```python
from build123d import *

# Parameters (mm, degrees)
F0_W     = 7.3944082856
F0_H     = 10
F0_W_2   = 7.394
F0_W_3   = 20
F0_H_2   = 5
F0_W_4   = 12.9295032024
F0_H_3   = 4
F0_W_5   = 4
F0_H_4   = 2
F1_DEPTH = 3


with BuildPart() as f1:
    # F0 (on Top) → F1 (new body)
    with BuildSketch(Plane.XY):
        with BuildLine():
            Line((72.3460563783, -23.3392287046), (-57.1586965515, -23.3392287046))
            Line((-57.1586965515, -23.3392287046), (-57.1586965515, -27.7934716308))
            Line((-57.1586965515, -27.7934716308), (-62.8714114428, -36.0010832548))
            Line((-62.8714114428, -36.0010832548), (-62.8714114428, -86.0010832548))
            ThreePointArc((-62.8714114428, -86.0010832548), (-61.102155393, -91.2274471391), (-56.5220229328, -94.3043828011))
            Line((-56.5220229328, -94.3043828011), (-46.5220229328, -94.3043828011))
            Line((-46.5220229328, -94.3043828011), (-39.6812242775, -101.5984539385))
            Line((-39.6812242775, -101.5984539385), (55.3187757225, -101.5984539385))
            Line((55.3187757225, -101.5984539385), (62.774033672, -94.9336862077))
            Line((62.774033672, -94.9336862077), (72.774033672, -94.9336862077))
            ThreePointArc((72.774033672, -94.9336862077), (76.135356085, -91.3724962002), (77.3572234082, -86.6303866614))
            Line((77.3572234082, -86.6303866614), (77.3572234082, -38.2830989705))
            Line((77.3572234082, -38.2830989705), (72.3460563783, -29.6293018271))
            Line((72.3460563783, -29.6293018271), (72.3460563783, -23.3392287046))
        make_face()
        Polygon((-33.379150033, -48.477938503), (-33.379150033, -46.477938503), (-34.9630750716, -46.477938503), (-34.9630750716, -50.477938503), (-33.379150033, -50.477938503), (-33.379150033, -60.477938503), (-34.9630750716, -60.477938503), (-34.9630750716, -64.477938503), (-33.379150033, -64.477938503), (-33.379150033, -66.477938503), (-49.892578274, -66.477938503), (-49.892578274, -64.477938503), (-47.892578274, -64.477938503), (-47.892578274, -60.477938503), (-49.892578274, -60.477938503), (-49.892578274, -50.477938503), (-47.892578274, -50.477938503), (-47.892578274, -46.477938503), (-49.892578274, -46.477938503), (-49.892578274, -44.477938503), (-45.951873064, -44.477938503), (-45.951873064, -42.477938503), (-47.4065802991, -42.477938503), (-47.4065802991, -40.477938503), (-34.9630750716, -40.477938503), (-31.379150033, -44.477938503), (-31.379150033, -48.477938503), align=None, mode=Mode.SUBTRACT)
        with Locations((-20.7225426286, -55.477938503)):
            Rectangle(F0_W, F0_H, mode=Mode.SUBTRACT)
        with Locations((-9.2900967939, -55.477938503)):
            Rectangle(F0_W_2, F0_H, mode=Mode.SUBTRACT)
        with BuildLine():
            Line((23.9428310841, -64.477938503), (23.9428310841, -36.0010832548))
            Line((23.9428310841, -36.0010832548), (33.941513979, -36.163380414))
            Line((33.941513979, -36.163380414), (33.941513979, -64.477938503))
            ThreePointArc((33.941513979, -64.477938503), (28.9421725316, -69.4772799505), (23.9428310841, -64.477938503))
        make_face(mode=Mode.SUBTRACT)
        with BuildLine():
            Line((38.3750386536, -64.477938503), (38.3750386536, -36.163380414))
            Line((38.3750386536, -36.163380414), (48.3750386536, -36.163380414))
            Line((48.3750386536, -36.163380414), (48.3750386536, -64.477938503))
            ThreePointArc((48.3750386536, -64.477938503), (43.3750386536, -69.477938503), (38.3750386536, -64.477938503))
        make_face(mode=Mode.SUBTRACT)
        with BuildLine():
            ThreePointArc((-28.9360948412, 27.1936530951), (-30.9919428027, 31.9537867139), (-28.9360948412, 36.7139203326))
            ThreePointArc((-28.9360948412, 36.7139203326), (-28.7221124747, 44.6950672996), (-36.7044586735, 44.8582988061))
            Line((-36.7044586735, 44.8582988061), (-62.5819294645, 29.6807988322))
            ThreePointArc((-62.5819294645, 29.6807988322), (-64.9426232399, 21.7216482709), (-57.1586965515, 18.8352252132))
            Line((-57.1586965515, 18.8352252132), (-57.1586965515, 13.1085557863))
            Line((-57.1586965515, 13.1085557863), (-57.1586965515, -11.8914442137))
            Line((-57.1586965515, -11.8914442137), (-57.1586965515, -23.3392287046))
            Line((-57.1586965515, -23.3392287046), (72.3460563783, -23.3392287046))
            Line((72.3460563783, -23.3392287046), (72.3460563783, 20.3706981729))
            ThreePointArc((72.3460563783, 20.3706981729), (77.602081112, 24.9911609789), (74.7467246428, 31.3803246156))
            Line((74.7467246428, 31.3803246156), (48.6460575227, 46.1706990491))
            Line((48.6460575227, 46.1706990491), (48.1593732874, 46.2963732235))
            ThreePointArc((48.1593732874, 46.2963732235), (40.4569849003, 43.1335810056), (42.8548762559, 35.1598642733))
            ThreePointArc((42.8548762559, 35.1598642733), (45.3786536259, 30.1186614419), (41.8995591407, 25.6825505592))
            Line((41.8995591407, 25.6825505592), (38.8500019908, 24.5999991894))
            Line((38.8500019908, 24.5999991894), (37.5105995638, 22.970316542))
            Line((37.5105995638, 22.970316542), (31.2569938554, 22.970316542))
            Line((31.2569938554, 22.970316542), (21.5923260851, 22.6860638537))
            Line((21.5923260851, 22.6860638537), (-9.1071914928, 22.6860638537))
            Line((-9.1071914928, 22.6860638537), (-15.6450517522, 22.6860638537))
            Line((-15.6450517522, 22.6860638537), (-23.319932078, 24.9601021238))
            Line((-23.319932078, 24.9601021238), (-28.9360948412, 27.1936530951))
        make_face()
        with BuildLine():
            ThreePointArc((-41.6760705411, -11.1311366782), (-46.2140015275, -7.0789042059), (-41.6760705411, -3.0266717337))
            Line((-41.6760705411, -3.0266717337), (-41.6760705411, -6.0266717337))
            ThreePointArc((-41.6760705411, -6.0266717337), (-43.1709154899, -7.0789042059), (-41.6760705411, -8.1311366782))
            Line((-41.6760705411, -8.1311366782), (-41.6760705411, -11.1311366782))
        make_face(mode=Mode.SUBTRACT)
        with BuildLine():
            Line((-39.6760705411, -6.0266717337), (-39.6760705411, -3.0266717337))
            ThreePointArc((-39.6760705411, -3.0266717337), (-34.941686368, -7.0789042059), (-39.6760705411, -11.1311366782))
            Line((-39.6760705411, -11.1311366782), (-39.6760705411, -8.1311366782))
            ThreePointArc((-39.6760705411, -8.1311366782), (-38.2074366729, -7.0789042059), (-39.6760705411, -6.0266717337))
        make_face(mode=Mode.SUBTRACT)
        Polygon((-41.6760705411, 10.8633437433), (-39.6760705411, 10.8633437433), (-39.6760705411, -1.3791318539), (-49.6760705411, -1.3791318539), (-49.6760705411, 10.8633437433), (-47.6760705411, 10.8633437433), (-47.6760705411, 0.6208681461), (-41.6760705411, 0.6208681461), (-41.6760705411, 4.5136589747), (-46.6760705411, 4.5136589747), (-46.6760705411, 6.5136589747), (-41.6760705411, 6.5136589747), align=None, mode=Mode.SUBTRACT)
        Polygon((-38.1764359772, 10.8633437433), (-36.1764359772, 10.8633437433), (-36.1764359772, 6.5136589747), (-31.1764359772, 6.5136589747), (-31.1764359772, 4.5136589747), (-33.379150033, 4.5136589747), (-36.1764359772, 4.5136589747), (-36.1764359772, -1.3791318539), (-38.1764359772, -1.3791318539), align=None, mode=Mode.SUBTRACT)
        Polygon((-10.0414280146, -10.3910174221), (-26.9197467715, -10.3910174221), (-26.9197467715, -4.3910174221), (-24.4197467715, -4.3910174221), (-24.4197467715, -8.3910174221), (-10.0414280146, -8.3910174221), align=None, mode=Mode.SUBTRACT)
        Polygon((-26.9197467715, 10.8633437433), (-20.9197467715, 10.8633437433), (-20.9197467715, 8.8633437433), (-24.4197467715, 8.8633437433), (-24.4197467715, 6.5136589747), (-21.9197467715, 6.5136589747), (-21.9197467715, 4.7421059447), (-24.4197467715, 4.7421059447), (-24.4197467715, 0.6208681461), (-20.9197467715, 0.6208681461), (-20.9197467715, -1.3791318539), (-26.9197467715, -1.3791318539), align=None, mode=Mode.SUBTRACT)
        Polygon((-17.0414280146, 10.8633437433), (-15.0414280146, 10.8633437433), (-15.0414280146, 6.5136589747), (-10.0414280146, 6.5136589747), (-10.0414280146, 4.5136589747), (-15.0414280146, 4.5136589747), (-15.0414280146, -1.3791318539), (-17.0414280146, -1.3791318539), align=None, mode=Mode.SUBTRACT)
        Polygon((-3.6023200955, -8.3910174221), (2.8300732374, -8.3910174221), (3.5192577634, -8.3910174221), (3.5192577634, 0), (5.5192577634, 0), (5.5192577634, -8.3910174221), (14.5462173969, -8.3910174221), (14.5462173969, -10.3910174221), (-3.6023200955, -10.3910174221), align=None, mode=Mode.SUBTRACT)
        Polygon((-3.6023200955, 0), (6.7411688089, 10.8633437433), (8.1896146413, 9.4842118894), (6.7411688089, 7.9629684176), (14.5462173969, 0), (13.1179118348, -1.3999797218), (5.3612146718, 6.5136589747), (-2.1538742631, -1.3791318539), align=None, mode=Mode.SUBTRACT)
        Polygon((18.9428310841, -1.3791318539), (18.9428310841, 10.8633437433), (20.9428310841, 10.8633437433), (20.9428310841, 0.7507229767), (28.9428310841, 0.6208681461), (28.9428310841, -1.3791318539), align=None, mode=Mode.SUBTRACT)
        Polygon((19.5553395897, -10.3910174221), (19.5553395897, -4.3910174221), (21.5553395897, -4.3910174221), (21.5553395897, -8.3910174221), (34.3452949524, -8.3910174221), (34.3452949524, -10.3910174221), align=None, mode=Mode.SUBTRACT)
        Polygon((32.3452949524, 10.8633437433), (34.3452949524, 10.8633437433), (34.3452949524, -1.3791318539), (32.3452949524, -1.3791318539), (32.3452949524, 2.3732802365), (29.2392894626, 2.3732802365), (29.2392894626, 4.3732802365), (32.3452949524, 4.3732802365), (32.3452949524, 7.1734678932), (29.2392894626, 7.1734678932), (29.2392894626, 9.1734678932), (32.3452949524, 9.1734678932), align=None, mode=Mode.SUBTRACT)
        Polygon((38.3750386536, -1.3791318539), (38.3750386536, 10.8633437433), (45.3750386536, 10.8633437433), (45.3750386536, 8.8633437433), (40.3750386536, 8.8633437433), (40.3750386536, 0.6208681461), (45.3750386536, 0.6208681461), (45.3750386536, -1.3791318539), align=None, mode=Mode.SUBTRACT)
        Polygon((38.3750386536, -10.3910174221), (38.3750386536, -4.3910174221), (40.3750386536, -4.3910174221), (40.3750386536, -8.3910174221), (56.2181740701, -8.3910174221), (56.2181740701, -10.3910174221), align=None, mode=Mode.SUBTRACT)
        Polygon((49.2181740701, -1.3791318539), (49.2181740701, 10.8633437433), (50.9630478919, 10.8633437433), (50.9630478919, 6.5136589747), (56.2181740701, 6.5136589747), (56.2181740701, 4.5136589747), (51.2181740701, 4.5136589747), (51.2181740701, -1.3791318539), align=None, mode=Mode.SUBTRACT)
        with Locations((6.2573329513, 15.6085557863)):
            Rectangle(F0_W_3, F0_H_2, mode=Mode.SUBTRACT)
        with BuildLine():
            Line((33.941513979, -36.163380414), (23.9428310841, -36.0010832548))
            Line((23.9428310841, -36.0010832548), (23.9428310841, -64.477938503))
            ThreePointArc((23.9428310841, -64.477938503), (28.9421725316, -69.4772799505), (33.941513979, -64.477938503))
            Line((33.941513979, -64.477938503), (33.941513979, -36.163380414))
        make_face()
        with BuildLine():
            Line((48.3750386536, -36.163380414), (38.3750386536, -36.163380414))
            Line((38.3750386536, -36.163380414), (38.3750386536, -64.477938503))
            ThreePointArc((38.3750386536, -64.477938503), (43.3750386536, -69.477938503), (48.3750386536, -64.477938503))
            Line((48.3750386536, -64.477938503), (48.3750386536, -36.163380414))
        make_face()
        Polygon((-33.379150033, -50.477938503), (-34.9630750716, -50.477938503), (-47.892578274, -50.477938503), (-49.892578274, -50.477938503), (-49.892578274, -60.477938503), (-47.892578274, -60.477938503), (-34.9630750716, -60.477938503), (-33.379150033, -60.477938503), align=None)
        with Locations((-41.4278266728, -48.477938503)):
            Rectangle(F0_W_4, F0_H_3)
        with Locations((-41.4278266728, -62.477938503)):
            Rectangle(F0_W_4, F0_H_3)
        Polygon((-34.9630750716, -42.477938503), (-33.379150033, -44.477938503), (-33.379150033, -46.477938503), (-33.379150033, -48.477938503), (-31.379150033, -48.477938503), (-31.379150033, -44.477938503), (-34.9630750716, -40.477938503), (-47.4065802991, -40.477938503), (-47.4065802991, -42.477938503), (-45.951873064, -42.477938503), (-41.951873064, -42.477938503), (-37.951873064, -42.477938503), align=None)
        Polygon((-33.379150033, -64.477938503), (-34.9630750716, -64.477938503), (-47.892578274, -64.477938503), (-49.892578274, -64.477938503), (-49.892578274, -66.477938503), (-33.379150033, -66.477938503), align=None)
        Polygon((-33.379150033, -46.477938503), (-33.379150033, -44.477938503), (-37.951873064, -44.477938503), (-41.951873064, -44.477938503), (-45.951873064, -44.477938503), (-49.892578274, -44.477938503), (-49.892578274, -46.477938503), (-47.892578274, -46.477938503), (-34.9630750716, -46.477938503), align=None)
        with Locations((-39.951873064, -43.477938503)):
            Rectangle(F0_W_5, F0_H_4)
        with Locations((-43.951873064, -43.477938503)):
            Rectangle(F0_W_5, F0_H_4)
        Polygon((-37.951873064, -44.477938503), (-33.379150033, -44.477938503), (-34.9630750716, -42.477938503), (-37.951873064, -42.477938503), align=None)
    extrude(amount=F1_DEPTH)


solid = f1.part
```
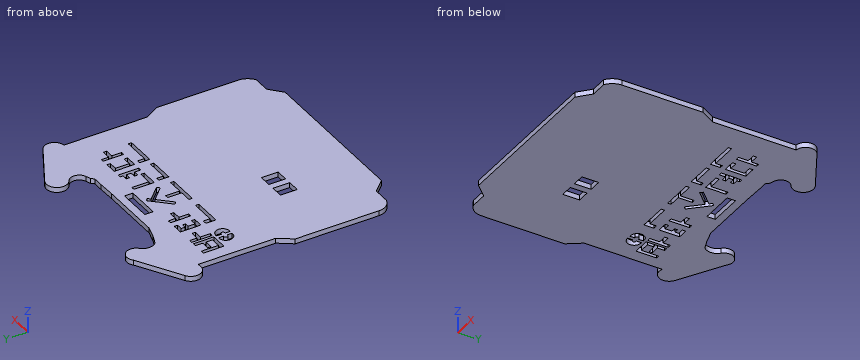
Input: part model. Units: mm. Frame: model coordinates. Give positions to 0.01 mm unless a question says otherwise; leave off trailing zeros. Order: outer loops, then holes, each group sorted by start corner. A loop starts at its lowest first (then second) coordinate and runs counter-clockwise, first axis right, second up. Notation, with made-up numbers: (2.25, 38) - (10.25, 38) arc R17 ccw to (10.25, 64) - close; hole circle Ø10 at (-26.5, 26). An arc over 180 degrees is marked (long way). Use a Markdown table: item, result.
(1) Section query B-B (y = -78). Output: boundary loops of the cut face in (x, z), then the cut area to 3 significant figures.
Computed values:
| item | result |
|---|---|
| outline | (-62.87, 0) - (77.36, 0) - (77.36, 3) - (-62.87, 3) - close |
| area | 421 mm2 |
(2) Section query C-C (z = 1.75). State how many separate pieces and enclosed holes the cut face has, then the cut area to 3 significant figures.
Computed values:
| item | result |
|---|---|
| separate pieces | 1 |
| enclosed holes | 18 |
| area | 16,900 mm2 |
(3) Pin query (flat end, axial travel): pin 1 (5 mm diameter, centred on x = 51.5, y = -86, fed in from -Z); pin 2 (0.9 mm diameter, centred on x = -21, z = 1.5, fed in from +Y); pin 3 (1.5 mm diameter, centred on y = 2.5, z = 2, fed in from +X); pin 4 (1.5 mm diameter, centred on y = 8.5, z = 1.5, fed in from -X). Return the tip coordinate at first contact, or that it passes through.
Computed values:
| item | result |
|---|---|
| pin 1 | stops at z = 0 |
| pin 2 | stops at y = 24.41 |
| pin 3 | stops at x = 72.35 |
| pin 4 | stops at x = -57.16 |
(4) Section query A-A (x = 10). Output: boundary loops of the cut face in (y, z), then the cut area to 3 significant figures.
Computed values:
| item | result |
|---|---|
| outline | (-101.6, 0) - (-10.39, 0) - (-10.39, 3) - (-101.6, 3) - close; (-8.39, 0) - (1.78, 0) - (1.78, 3) - (-8.39, 3) - close; (4.64, 0) - (13.11, 0) - (13.11, 3) - (4.64, 3) - close; (18.11, 0) - (22.69, 0) - (22.69, 3) - (18.11, 3) - close |
| area | 343 mm2 |
(5) Line query: line 1 (X direction, y = -54.5, z = 1.2); line 2 (Y direction, x = 22.5, z = 0.2); line 3 (Y direction, x = -24, z = 1.45). Output: solid intervals per line, ascending. Write a range as from..to.
Computed values:
| item | result |
|---|---|
| line 1 | x = -62.87..-24.42, -17.03..-12.99, -5.59..77.36 |
| line 2 | y = -101.6..-10.39, -8.39..-1.38, 0.73..22.71 |
| line 3 | y = -101.6..-60.48, -50.48..-10.39, -8.39..-1.38, 0.62..4.74, 6.51..8.86, 10.86..25.23 |
(6) Section query D-D (y = -13). Output: boundary loops of the cut face in (x, z).
Computed values:
| item | result |
|---|---|
| outline | (-57.16, 0) - (72.35, 0) - (72.35, 3) - (-57.16, 3) - close |
